Could you check a few things on this model? Use its own coordinates, in mm. Round coordinates to 2 decimals unless told otherwise and drop trailing zeros. Write each loop counter-clockwise with the first axis right and the second up, starting at its lowest first coordinate (ties: lowest second). Pieces come first, ordered by that corner, then holes.
```python
from build123d import *

# Parameters (mm, degrees)
F0_W     = 38.1
F0_H     = 19.05
F1_DEPTH = 38.1
F4_D     = 10.71626
F4_DEPTH = 38.1
F4_TIP   = 3.2194893086
F5_D     = 12.7


# Not quite as in the source:
# - a length typed as a fraction of an inch, garbled in the dataset ("3 / 203.2 mm" for 3/8 in), is restored


with BuildPart() as f1:
    # F0 (on Front) → F1 (new body, symmetric)
    with BuildSketch(Plane.XZ):
        Rectangle(F0_W, F0_H)
    extrude(amount=F1_DEPTH, both=True)

    # F4
    with Locations(Plane.XZ.offset(38.1)):
        with Locations((0, 0)):
            Hole(F4_D / 2, depth=F4_DEPTH)
            with Locations((0, 0, -(F4_DEPTH + F4_TIP / 2))):  # 118° drill point
                Cone(0, F4_D / 2, F4_TIP, mode=Mode.SUBTRACT)

    # F5 (through all)
    with Locations(Plane.YZ.offset(19.05)):
        with Locations((25.4, 0)):
            Hole(F5_D / 2)


solid = f1.part
```
Q1. I'm going to push flat-ended pins straight in: pin 1 Ø1 at (x, z) = (3, -1) entering from -Y; pin 2 Ø5 at (x, z) = (-2, 2.5) entering from -Y. Where does each tip first touch, or does it pass through?
Q2. If I drill on L1, parallel to Z at x = 0, y = -18.5 (3 decimals); L2, parallel to X at y = -26, z = 2; L3, parallel to X at y = -28.5, z = 0, over which ranges is the centre line in solid material (lowest first)?
Q3. Imagine slicing it at B-B, the plane x = -11. Write out the boundary of the cut face in (y, z) (3 decimals), then the cut area to 3 significant figures.
Q4. Imagine slicing it at A-A, the plane y = 25.4. Write out the boundary of the cut face in (x, z) (3 decimals).
Q5. Imagine slicing it at C-C, the plane y = -33. Write out the boundary of the cut face in (x, z) (3 decimals).
Q6. We'd pull the mould along X, two halves only. Please class faces 1 (the flat face through (-19.05, -1, 0)), 2 (the flat face through (19.05, -1, 0)), 3 (the flat face through (4, -38.1, 4)), 4 (the cylindrical face through (-2.472, -18.783, -4.754)): pulls with the +X half, pulls with the -X half, needs draft (parallel to the pull), parting line crosses it, or undercut.
Results found:
1. pin 1: stops at y = 1.02
1. pin 2: stops at y = -38.1
2. L1: z = -9.525 to -5.358, 5.358 to 9.525
2. L2: x = -19.05 to -4.97, 4.97 to 19.05
2. L3: x = -19.05 to -5.36, 5.36 to 19.05
3. outline: (-38.1, -9.525) - (38.1, -9.525) - (38.1, 9.525) - (-38.1, 9.525) - close; hole circle Ø12.7 at (25.4, 0)
3. area: 1,320 mm2
4. outline: (-19.05, -9.525) - (19.05, -9.525) - (19.05, -6.35) - (-19.05, -6.35) - close; (-19.05, 6.35) - (19.05, 6.35) - (19.05, 9.525) - (-19.05, 9.525) - close
5. outline: (-19.05, -9.525) - (19.05, -9.525) - (19.05, 9.525) - (-19.05, 9.525) - close; hole circle Ø10.716 at (0, 0)
6. face 1: pulls with the -X half
6. face 2: pulls with the +X half
6. face 3: needs draft
6. face 4: undercut
